from build123d import *

# Parameters (mm, degrees)
BOSS_EXTRUDE2_DEPTH      = 1
BOSS_EXTRUDE2_DEPTH_BACK = 2
SKETCH1_R                = 0.15
SKETCH5_R                = 0.15
BOSS_EXTRUDE3_DEPTH      = 0.5
BOSS_EXTRUDE4_DEPTH      = 7
BOSS_EXTRUDE4_DEPTH_BACK = 2
SKETCH6_R                = 0.15
SKETCH16_R               = 0.15


with BuildPart() as part:
    # Sketch1 → Boss-Extrude2 (new, two sides: drawn at the far end of the back side and taken through both)
    with BuildSketch(Plane.XY.offset(-BOSS_EXTRUDE2_DEPTH_BACK)):
        Circle(SKETCH1_R)
    extrude(amount=BOSS_EXTRUDE2_DEPTH + BOSS_EXTRUDE2_DEPTH_BACK)

    # Sketch4 → Revolve2 (revolve)
    with BuildSketch(Plane(origin=(0, 0, 0), x_dir=(0, 0, -1), z_dir=(1, 0, 0))):
        with BuildLine():
            ThreePointArc((-3.699926528, 1.261319774), (-3.380844772, 1.292746584), (-3.074025149, 1.385819299))
            ThreePointArc((-3.074025149, 1.385819299), (-1.730128131, 1.287360597), (-1.007518844, 0.15))
            Line((-1.007518844, 0.15), (-1, 0.15))
            Line((-1, 0.15), (-1, 0))
            Line((-1, 0), (-2.5, 0))
            Line((-2.5, 0), (-4, 0))
            Line((-4, 0), (-11.5, 0))
            Line((-11.5, 0), (-13, 0))
            Line((-13, 0), (-13, 0.15))
            Line((-13, 0.15), (-12.992481156, 0.15))
            ThreePointArc((-12.992481156, 0.15), (-12.269871869, 1.287360597), (-10.925974851, 1.385819299))
            ThreePointArc((-10.925974851, 1.385819299), (-10.619155228, 1.292746584), (-10.300073472, 1.261319774))
            Line((-10.300073472, 1.261319774), (-3.699926528, 1.261319774))
        make_face()
    revolve(axis=Axis((0, 0, 4), (0, 0, 1)))

    # Sketch5 → Boss-Extrude3 (add)
    with BuildSketch(Plane.XY.offset(13)):
        Circle(SKETCH5_R)
    extrude(amount=BOSS_EXTRUDE3_DEPTH)



with BuildPart() as body_2:
    # Sketch6 → Boss-Extrude4 (new, two sides: drawn at the far end of the back side and taken through both)
    with BuildSketch(Plane.XY.offset(-BOSS_EXTRUDE4_DEPTH_BACK)):
        with Locations((4, 0)):
            Circle(SKETCH6_R)
    extrude(amount=BOSS_EXTRUDE4_DEPTH + BOSS_EXTRUDE4_DEPTH_BACK)


with BuildPart() as part_1:
    add(part.part)

    add(body_2.part)  # Sweep3 merges body 2
    # Sweep3: sweep along a path in Sketch7
    with BuildLine(Plane(origin=(0, 0, 0), x_dir=(1, 0, 0), z_dir=(0, 1, 0))) as sweep3_path:
        ThreePointArc((4.15, -7), (4.134550157, -7.156464216), (4.088797373, -7.306885063))
        Line((4.088797373, -7.306885063), (1.388797373, -13.806885063))
        ThreePointArc((1.388797373, -13.806885063), (0.493535784, -14.284550157), (-0.15, -13.5))
    # Sketch16 → Sweep3 (sweep)
    with BuildSketch(Plane.XY.offset(7)):
        with Locations((4, 0)):
            Circle(SKETCH16_R)
    sweep(path=sweep3_path.line)


solid = part_1.part
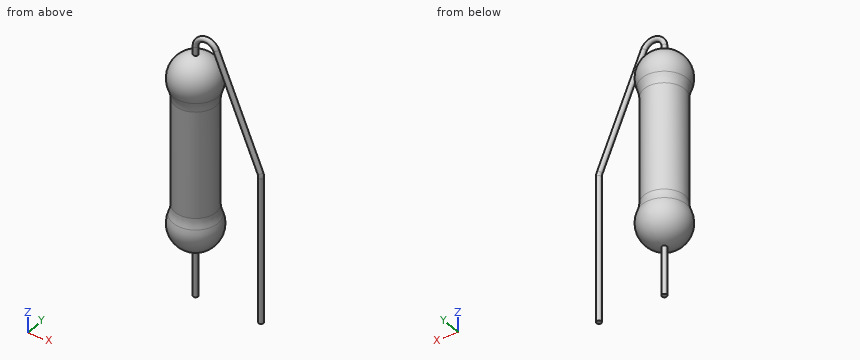
Can you work these out from the model? Positions are in its coordinate system, mm. Coordinates: 2 decimals unless noted, no trailing zeros. Loops run counter-clockwise (first coordinate to the right, second up) from the corner with the lowest first, then second, coordinate; pieces in that order, holes last. Notation, with made-up numbers: (46, 61.25) - (75, 61.25) arc R19 ccw to (75, 69.25) - close; hole circle Ø3 at (59.25, -20). An arc over 180 degrees is marked (long way). Put each result on its own line as item: value. Start each with the question number.
Item 1: For pin 1 (1.5 mm diameter, centred on x = 1.5, z = 3.5, fed in from +Y); pin 2 (1 mm diameter, centred on x = -0.5, z = 7.5, fed in from -Y), each with a flat end and sliding along its axis, tell me the tip position at first contact or that it passes through.
Item 2: If I drill on line 1 along Y through (x, z) = (0, -0.25); line 2 along Y through (x, z) = (0.05, 6); line 3 along Z through (x, y) = (1, -1), over which ranges is the centre line in solid material (lowest first)?
Item 3: Suppose I cut it at A-A (z = 6.5). Please give me the cut outline in (x, y).
Here are the results:
1. pin 1: y = 1.07
1. pin 2: y = -1.26
2. line 1: -0.15 to 0.15
2. line 2: -1.26 to 1.26
2. line 3: 2 to 3, 11 to 12
3. outline: circle Ø2.52 at (0, 0); circle Ø0.3 at (4, 0)
